The model under review builds one solid part; all positions refer to its coordinate system, in mm. Give positions to 0.01 mm unless a question says otherwise; leave off trailing zeros. Order: outer loops, then holes, each group sorted by start corner. A loop starts at its lowest first (then second) coordinate and runs counter-clockwise, first axis right, second up.
```python
from build123d import *

# Parameters (mm, degrees)
F0_R     = 13.855
F0_R_2   = 1
F1_DEPTH = 2.6
F2_R     = 0.15
F3_SIZE  = 0.25


with BuildPart() as f1:
    # F0 (on Top) → F1 (new body)
    with BuildSketch(Plane.XY):
        Circle(F0_R)
        with Locations((-6, -3.475305)):
            Circle(F0_R_2, mode=Mode.SUBTRACT)
        with Locations((6, -3.475305)):
            Circle(F0_R_2, mode=Mode.SUBTRACT)
        with Locations((0, 6.917)):
            Circle(F0_R_2, mode=Mode.SUBTRACT)
    extrude(amount=F1_DEPTH)

    # F2
    f2_edges = [f1.edges().sort_by_distance(p)[0] for p in [
        (-13.855, 0, 2.6),
        (-13.855, 0, 0),
    ]]
    fillet(f2_edges, radius=F2_R)

    # F3
    f3_edges = [f1.edges().sort_by_distance(p)[0] for p in [
        (-1, 6.917, 2.6),
        (5, -3.475305, 2.6),
        (5, -3.475305, 0),
        (-1, 6.917, 0),
        (-7, -3.475305, 2.6),
        (-7, -3.475305, 0),
    ]]
    chamfer(f3_edges, length=F3_SIZE)


solid = f1.part
```
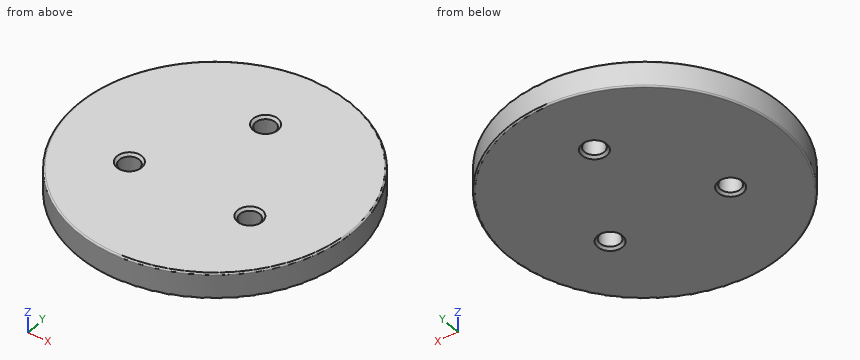
Item 1: Take a section at A-A (x = 0). Give the boundary of the cut face in (y, z) (3 decimals).
Values found:
outline: (-13.855, 0.15) arc R0.15 ccw to (-13.705, 0) - (5.667, 0) - (5.917, 0.25) - (5.917, 2.35) - (5.667, 2.6) - (-13.705, 2.6) arc R0.15 ccw to (-13.855, 2.45) - close; (7.917, 0.25) - (8.167, 0) - (13.705, 0) arc R0.15 ccw to (13.855, 0.15) - (13.855, 2.45) arc R0.15 ccw to (13.705, 2.6) - (8.167, 2.6) - (7.917, 2.35) - close
Item 2: For line 1 (X direction, y = -4.5, z = 2.55); line 2 (X direction, y = -3.25, z = 1.35); line 3 (Y direction, x = 5.5, z = 1.25), list the stretches that pass through material, from the lowest coordinate up.
Values found:
line 1: x = -13.06 to -6.62, -5.38 to 5.38, 6.62 to 13.06
line 2: x = -13.47 to -6.97, -5.03 to 5.03, 6.97 to 13.47
line 3: y = -12.72 to -4.34, -2.61 to 12.72
Item 3: Clearance check with a flat-ended pin moving along its axis: pin 1 Ø1.6 at (x, y) = (-6, -3.48) entering from +Z. State where the tip first meets the part, or that it passes through.
Values found:
pin 1: passes through
Item 4: Take a section at B-B (z = 1.65). Give the boundary of the cut face in (x, y) (3 decimals), and give its area (3 significant figures).
Values found:
outline: circle Ø27.71 at (0, 0); hole circle Ø2 at (-6, -3.475); hole circle Ø2 at (0, 6.917); hole circle Ø2 at (6, -3.475)
area: 594 mm2
